Verification items for the finished model (mm, model axes). A direction names the side the tool comes from. Give positions to 0.01 mm unless a question says otherwise; leave off trailing zeros. Write each loop counter-clockwise with the first axis right and the second up, starting at its lowest first coordinate (ties: lowest second). Pieces come first, ordered by that corner, then holes. Notation, with made-up numbers: (1, 69) -> (10, 69) arc R20 ccw to (10, 81) -> close; hole circle Ø8 at (0.5, 25.25). An arc over 180 degrees is marked (long way). Answer as CSV lines item,"result". Start each with the question number.
1) Sectioned sample at D-D on z = 1.65. Record the cut outline in (x, y), and give its area (3 significant figures).
2) Sectioned sample at B-B on y = -15. Record the cut outline in (x, z).
3) Sectioned sample at C-C on x = -22. Record the cut outline in (y, z).
4) Sectioned sample at A-A on x = 7.5. Record the cut outline in (y, z), and give its area (3 significant figures).
5) Mould release check, pull along X, two halves, no side actions. Record for faces 4 (the cylindrical face through (0.14, 35.208, 1.972)), 5 (the cylindrical face through (-23.45, -13.77, 1.97)), 6 (the flat face through (-1, -14, 4)): released by +X, released by -X, zero draft, split by the parting line, or undercut.
6) Tool access check on faces 1 (the flat face through (-1, -14, 0)), 2 (the flat face through (0, -26.786, 2)), 3 (the flat face through (-7.2, -1.694, 1.972)). Record the directions out of +Z, -Z, +X, -X, +Y, -Y that give a thin tool (end or side, any length) a straight path to the whole face; none if there is none.
7) Gauge pin test, flat ends, axial feed: pin 1 Ø9 at (x, y) = (-22.79, -18.76) entering from -Z; pin 2 Ø1.5 at (x, z) = (12, 0.5) entering from +Y; pin 3 Ø2 at (x, z) = (15.5, 2) entering from -Y. Record the tip position at first contact, or that the pin passes through.
8) Material ranges on L1, parallel to X at y = -19, z = 2; L2, parallel to Y at x = -6, z = 2.45; L3, parallel to X at y = -15.5, z = 3.05, recorded low to high.
```python
from build123d import *

# Parameters (mm, degrees)
SKETCH_1_R      = 9.53
SKETCH_1_R_2    = 5.03
EXTRUDE_1_DEPTH = 4


with BuildPart() as part:
    # 草图1 → 凸台-拉伸1 (new body)
    with BuildSketch(Plane.XY):
        with BuildLine():
            Line((-18.494622549, 4.742999843), (-23.409453688, -3.769737399))
            ThreePointArc((-23.409453688, -3.769737399), (-35.781809628, -26.257000157), (-10.121090849, -26.785856986))
            Line((-10.121090849, -26.785856986), (-0.291428571, -26.785856986))
            Line((-0.291428571, -26.785856986), (9.538233706, -26.785856986))
            ThreePointArc((9.538233706, -26.785856986), (35.198952485, -26.257000157), (22.826596545, -3.769737399))
            Line((22.826596545, -3.769737399), (17.911765406, 4.742999843))
            Line((17.911765406, 4.742999843), (12.996934268, 13.255737086))
            ThreePointArc((12.996934268, 13.255737086), (-0.291428571, 35.214143014), (-13.579791411, 13.255737086))
            Line((-13.579791411, 13.255737086), (-18.494622549, 4.742999843))
        make_face()
        with Locations((-0.291428571, 20.214143014)):
            Circle(SKETCH_1_R, mode=Mode.SUBTRACT)
        with Locations((22.208571429, -18.757000157)):
            Circle(SKETCH_1_R_2, mode=Mode.SUBTRACT)
        with Locations((-22.791428571, -18.757000157)):
            Circle(SKETCH_1_R_2, mode=Mode.SUBTRACT)
        with BuildLine():
            Line((9.268171867, -6.285856986), (4.038698447, 2.771856673))
            ThreePointArc((4.038698447, 2.771856673), (-0.291428571, 5.271856673), (-4.62155559, 2.771856673))
            Line((-4.62155559, 2.771856673), (-9.85102901, -6.285856986))
            ThreePointArc((-9.85102901, -6.285856986), (-9.85102901, -11.285856986), (-5.520901991, -13.785856986))
            Line((-5.520901991, -13.785856986), (4.938044848, -13.785856986))
            ThreePointArc((4.938044848, -13.785856986), (9.268171867, -11.285856986), (9.268171867, -6.285856986))
        make_face(mode=Mode.SUBTRACT)
    extrude(amount=EXTRUDE_1_DEPTH)


solid = part.part
```
Ans:
1,outline,"(-23.41, -3.77) arc R15 ccw (long way) to (-10.12, -26.79) -> (9.54, -26.79) arc R15 ccw (long way) to (22.83, -3.77) -> (13, 13.26) arc R15 ccw (long way) to (-13.58, 13.26) -> close; hole circle Ø10.06 at (-22.79, -18.76); hole (-9.85, -6.29) arc R5 ccw to (-5.52, -13.79) -> (4.94, -13.79) arc R5 ccw to (9.27, -6.29) -> (4.04, 2.77) arc R5 ccw to (-4.62, 2.77) -> close; hole circle Ø19.06 at (-0.29, 20.21); hole circle Ø10.06 at (22.21, -18.76)"
1,area,"2,310 mm²"
2,outline,"(-37.31, 0) -> (-26.14, 0) -> (-26.14, 4) -> (-37.31, 4) -> close; (-19.45, 0) -> (18.86, 0) -> (18.86, 4) -> (-19.45, 4) -> close; (25.55, 0) -> (36.73, 0) -> (36.73, 4) -> (25.55, 4) -> close"
3,outline,"(-33.74, 0) -> (-23.72, 0) -> (-23.72, 4) -> (-33.74, 4) -> close; (-13.79, 0) -> (-1.33, 0) -> (-1.33, 4) -> (-13.79, 4) -> close"
4,outline,"(-26.79, 0) -> (-13.08, 0) -> (-13.08, 4) -> (-26.79, 4) -> close; (-3.22, 0) -> (14.73, 0) -> (14.73, 4) -> (-3.22, 4) -> close; (25.7, 0) -> (33.03, 0) -> (33.03, 4) -> (25.7, 4) -> close"
4,area,"156 mm²"
5,face 4,"split by the parting line"
5,face 5,"undercut"
5,face 6,"zero draft"
6,face 1,"-Z, +X, -X, +Y, -Y"
6,face 2,"+Z, -Z, -Y"
6,face 3,"+Z, -Z"
7,pin 1,"passes through"
7,pin 2,"stops at y = 29.8"
7,pin 3,"stops at y = -32.63"
8,L1,"x = -37.79 to -27.82, -17.77 to 17.18, 27.23 to 37.21"
8,L2,"y = -26.79 to -13.76, 0.38 to 12.58, 27.85 to 34.09"
8,L3,"x = -37.43 to -26.62, -18.96 to 18.38, 26.04 to 36.85"
